Part model, mm, in its own coordinate system. A direction names the side the tool comes from. Round coordinates to 2 decimals unless told otherwise and drop trailing zeros. Loops run counter-clockwise (first coordinate to the right, second up) from the corner with the lowest first, then second, coordinate; pieces in that order, holes last.
1) Band-saw the part on A-A, the plane x = 31.5. Write the cut outline in (y, z), then the cut area to 4 significant figures.
2) 3-axis set-ups, long thin cutter, end or side, ignore diameter. For faces 1 (the flat face through (1, 0, 0)), 2 (the flat face through (-5.63, 0.8, -16.56)): which of +Z, -Z, +X, -X, +Y, -Y reach the whole face in a straight line?
3) Band-saw the part on D-D, the plane x = 0. Write the cut outline in (y, z).
4) Mould opens along X. For faces 3 (the flat face through (-15, 0.5, -19)), 4 (the cylindrical face through (42.18, 0.54, 26.15)), 5 (the flat face through (-6.8, 0.5, -18.2)), 6 (the cylindrical face through (-42.15, 0.54, 26.18)) say: +X half, -X half, draft (parallel to the pull), parting line (faces both ways), or undercut.
5) Band-saw the part on B-B, the plane y = 0.7. State how many separate pieces and enclosed holes the cut face has, then the cut area to 3 significant figures.
6) Probe line 1 (Z direction, x = 10, y = 0.95); line 2 (Z direction, x = -36, y = 0.8); line 3 (X direction, y = 0.75, z = 4). List the from-to ranges inside material, lowest first.
7) Drop a flat-ended pin along its axis: P1, Ø2, axis at x = 2.5, z = -19, coming from the -Y side. Give the stop position or say it passes through.
8) Band-saw the part on C-C, the plane z = 11. Write the cut outline in (x, y).
from build123d import *

# Parameters (mm, degrees)
EXTRUDE_1_DEPTH     = 1.1
SKETCH_4_R          = 12.96
SKETCH_4_W          = 5.084081154
SKETCH_4_H          = 7
SKETCH_4_W_2        = 3.808622708
SKETCH_4_H_2        = 5.930745221
SKETCH_4_W_3        = 1.586812329
SKETCH_4_H_3        = 1.62095201
CUT_EXTRUDE_8_DEPTH = 0.6
CUT_EXTRUDE_9_DEPTH = 51.441401646


with BuildPart() as part:
    # Эскиз1 → Бобышка-Вытянуть1 (new body)
    with BuildSketch(Plane(origin=(0, 0, 0), x_dir=(1, 0, 0), z_dir=(0, 1, 0))):
        with BuildLine():
            Line((-40.75, 26.75), (40.75, 26.75))
            ThreePointArc((40.75, 26.75), (42.164213562, 26.164213562), (42.75, 24.75))
            Line((42.75, 24.75), (42.75, -24.75))
            ThreePointArc((42.75, -24.75), (42.164213562, -26.164213562), (40.75, -26.75))
            Line((40.75, -26.75), (-40.75, -26.75))
            ThreePointArc((-40.75, -26.75), (-42.164213562, -26.164213562), (-42.75, -24.75))
            Line((-42.75, -24.75), (-42.75, 24.75))
            ThreePointArc((-42.75, 24.75), (-42.164213562, 26.164213562), (-40.75, 26.75))
        make_face()
    extrude(amount=EXTRUDE_1_DEPTH)

    # Эскиз4 → Вырез-Вытянуть8 (cut)
    # profile 1 of 9: a face of its own
    with BuildSketch(Plane(origin=(0, 1.1, 0), x_dir=(1, 0, 0), z_dir=(0, 1, 0))):
        with Locations(Location((0, -7.603080064, 0), (0, 0, 270))):
            Circle(SKETCH_4_R)
    # profile 2 of 9: a face of its own
    with BuildSketch(Plane(origin=(0, 1.1, 0), x_dir=(1, 0, 0), z_dir=(0, 1, 0))):
        Polygon((-23.824034335, 14.987763796), (-28.831642606, 14.987763796), (-28.831642606, 21.915387674), (-28.193913383, 21.915387674), (-28.193913383, 15.520342805), (-23.824034335, 15.520342805), align=None)
    # profile 3 of 9: a face of its own
    with BuildSketch(Plane(origin=(0, 1.1, 0), x_dir=(1, 0, 0), z_dir=(0, 1, 0))):
        with Locations((-19.559988295, 18.487763796)):
            Rectangle(SKETCH_4_W, SKETCH_4_H)
        with Locations((-19.559988295, 18.485715415)):
            Rectangle(SKETCH_4_W_2, SKETCH_4_H_2, mode=Mode.SUBTRACT)
    # profile 4 of 9: a face of its own
    with BuildSketch(Plane(origin=(0, 1.1, 0), x_dir=(1, 0, 0), z_dir=(0, 1, 0))):
        Polygon((-10.265119001, 16.274146941), (-11.591104175, 14.987763796), (-14.095591104, 14.987763796), (-15.372415139, 16.215426691), (-15.372415139, 20.747810616), (-14.094225517, 21.987763796), (-11.593835349, 21.987763796), (-10.265119001, 20.691821541), (-10.677526336, 20.347693566), (-11.875146313, 21.451088026), (-13.819742489, 21.451088026), (-14.734685915, 20.562090757), (-14.734685915, 16.405243312), (-13.819742489, 15.520342805), (-11.872415139, 15.520342805), (-10.677526336, 16.618274916), align=None)
    # profile 5 of 9: a face of its own
    with BuildSketch(Plane(origin=(0, 1.1, 0), x_dir=(1, 0, 0), z_dir=(0, 1, 0))):
        Polygon((-3.535505267, 15.305945614), (-3.947912602, 14.960452052), (-7.36597737, 18.213280768), (-8.005072181, 18.213280768), (-8.005072181, 15.056043156), (-8.642801405, 15.056043156), (-8.642801405, 21.915387674), (-8.005072181, 21.915387674), (-8.005072181, 18.754053301), (-7.363246196, 18.754053301), (-3.947912602, 22.01507554), (-3.535505267, 21.664119629), (-6.823839251, 18.485032622), align=None)
    # profile 6 of 9: a face of its own
    with BuildSketch(Plane(origin=(0, 1.1, 0), x_dir=(1, 0, 0), z_dir=(0, 1, 0))):
        Polygon((3.094420601, 14.987763796), (-1.913187671, 14.987763796), (-1.913187671, 21.987763796), (3.094420601, 21.987763796), (3.094420601, 21.451088026), (-1.275458447, 21.451088026), (-1.275458447, 18.754053301), (0.872610222, 18.754053301), (0.872610222, 18.213280768), (-1.275458447, 18.213280768), (-1.275458447, 15.520342805), (3.094420601, 15.520342805), align=None)
    # profile 7 of 9: a face of its own
    with BuildSketch(Plane(origin=(0, 1.1, 0), x_dir=(1, 0, 0), z_dir=(0, 1, 0))):
        Polygon((9.900507218, 19.480545692), (8.595005853, 18.213280768), (6.825204838, 18.213280768), (9.923722201, 15.305945614), (9.511314865, 14.960452052), (6.093250098, 18.213280768), (5.454155287, 18.213280768), (5.454155287, 15.056043156), (4.816426063, 15.056043156), (4.816426063, 21.987763796), (8.593640265, 21.987763796), (9.900507218, 20.719133285), align=None)
        Polygon((9.262777995, 19.671727901), (9.262777995, 20.532047838), (8.312329302, 21.451088026), (5.454155287, 21.451088026), (5.454155287, 18.754053301), (8.316426063, 18.754053301), align=None, mode=Mode.SUBTRACT)
    # profile 8 of 9: a face of its own
    with BuildSketch(Plane(origin=(0, 1.1, 0), x_dir=(1, 0, 0), z_dir=(0, 1, 0))):
        Polygon((23.283261803, 17.141294815), (22.246781116, 17.141294815), (22.246781116, 15.056043156), (21.609051892, 15.056043156), (21.609051892, 17.141294815), (20.022239563, 17.141294815), (20.022239563, 15.056043156), (19.388607101, 15.056043156), (19.388607101, 17.141294815), (18.348029653, 17.141294815), (18.348029653, 17.672508236), (19.388607101, 17.672508236), (19.388607101, 19.293460246), (18.348029653, 19.293460246), (18.348029653, 19.835598365), (19.388607101, 19.835598365), (19.388607101, 21.915387674), (20.022239563, 21.915387674), (20.022239563, 19.835598365), (21.609051892, 19.835598365), (21.609051892, 21.915387674), (22.246781116, 21.915387674), (22.246781116, 19.835598365), (23.283261803, 19.835598365), (23.283261803, 19.293460246), (22.246781116, 19.293460246), (22.246781116, 17.672508236), (23.283261803, 17.672508236), align=None)
        with Locations((20.815645728, 18.482984241)):
            Rectangle(SKETCH_4_W_3, SKETCH_4_H_3, mode=Mode.SUBTRACT)
    # profile 9 of 9: a face of its own
    with BuildSketch(Plane(origin=(0, 1.1, 0), x_dir=(1, 0, 0), z_dir=(0, 1, 0))):
        Polygon((28.97639485, 16.244104022), (27.673624659, 14.987763796), (26.282091299, 14.987763796), (25.005267265, 16.215426691), (25.005267265, 20.747810616), (26.283456886, 21.987763796), (27.669527897, 21.987763796), (28.97639485, 20.719133285), align=None)
        Polygon((28.338665626, 16.432555056), (28.338665626, 20.533413426), (27.395044869, 21.451088026), (26.557939914, 21.451088026), (25.642996488, 20.562090757), (25.642996488, 16.405243312), (26.557939914, 15.520342805), (27.397776044, 15.520342805), align=None, mode=Mode.SUBTRACT)
    extrude(amount=-CUT_EXTRUDE_8_DEPTH, mode=Mode.SUBTRACT)

    # Эскиз5 → Вырез-Вытянуть9 (cut, through all)
    with BuildSketch(Plane(origin=(0, 1.1, 0), x_dir=(1, 0, 0), z_dir=(0, 1, 0))):
        with BuildLine():
            Line((-35.845264221, 10.897827852), (35.845264221, 10.897827852))
            ThreePointArc((35.845264221, 10.897827852), (36.845264221, 9.897827852), (35.845264221, 8.897827852))
            Line((35.845264221, 8.897827852), (-35.845264221, 8.897827852))
            ThreePointArc((-35.845264221, 8.897827852), (-36.845264221, 9.897827852), (-35.845264221, 10.897827852))
        make_face()
    extrude(amount=-CUT_EXTRUDE_9_DEPTH, mode=Mode.SUBTRACT)


solid = part.part
Reported:
1. outline: (0, -26.75) - (1.1, -26.75) - (1.1, -10.9) - (0, -10.9) - close; (0, -8.9) - (1.1, -8.9) - (1.1, 26.75) - (0, 26.75) - close
1. area: 56.65 mm2
2. face 1: +Z, -Z, +X, -X, -Y
2. face 2: +Y
3. outline: (0, -26.75) - (1.1, -26.75) - (1.1, -21.99) - (0.5, -21.99) - (0.5, -21.45) - (1.1, -21.45) - (1.1, -18.75) - (0.5, -18.75) - (0.5, -18.21) - (1.1, -18.21) - (1.1, -15.52) - (0.5, -15.52) - (0.5, -14.99) - (1.1, -14.99) - (1.1, -10.9) - (0, -10.9) - close; (0, -8.9) - (1.1, -8.9) - (1.1, -5.36) - (0.5, -5.36) - (0.5, 20.56) - (1.1, 20.56) - (1.1, 26.75) - (0, 26.75) - close
4. face 3: undercut
4. face 4: +X half
4. face 5: undercut
4. face 6: -X half
5. separate pieces: 5
5. enclosed holes: 10
5. area: 3,810 mm2
6. line 1: z = -26.75 to -10.9, -8.9 to -0.64, 15.85 to 26.75
6. line 2: z = -26.75 to -10.89, -8.91 to 26.75
6. line 3: x = -42.75 to -12.45, 12.45 to 42.75
7. P1: stops at y = 0
8. outline: (-42.75, 0) - (42.75, 0) - (42.75, 1.1) - (12.51, 1.1) - (12.51, 0.5) - (-12.51, 0.5) - (-12.51, 1.1) - (-42.75, 1.1) - close
